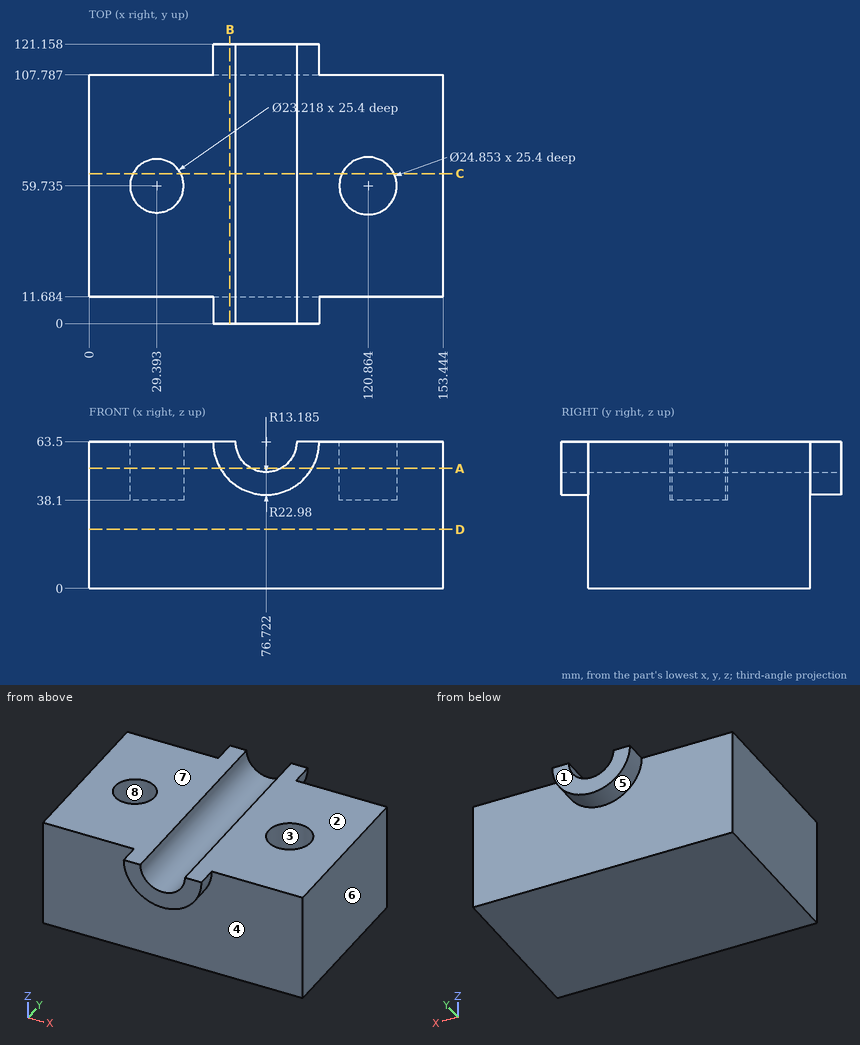
Could you check a few things on this drawing? It's one solid part, dimensions in mm from its lowest x, y, z. A direction names the side the tool comes from. Coordinates: 2 decimals unless noted, no trailing zeros. Write each loop counter-clockwise with the first axis right and the second up, starting at its lowest first coordinate (ties: lowest second). Pieces come first, ordered by that corner, then holes. Notation, with made-up numbers: (-30.75, -4) - (18.25, -4) arc R17 cw to (18.25, 5) - close; hole circle Ø7 at (54, 65.5). An arc over 180 degrees is marked (long way). Return JSON: item names as keys, results as strings. Group by question number.
Item 1: I'm going to push flat-ended pins straight in: pin 1 Ø1 at (y, z) = (35.5, 56) entering from -X; pin 2 Ø8 at (x, z) = (35.5, 25.5) entering from +Y; pin 3 Ø1.5 at (x, z) = (57.5, 38.5) entering from -Y. Where does each tip first touch, or does it pass through?
Item 2: Which directions (+Z, -Z, +X, -X, +Y, -Y) give clear straight access to the entire face, cutting with the end or side of a thin tool? Please do the marked faces 4, 5, 6, 7 and 8.
Item 3: We'd pull the mould along Y, two halves only. Please class the marked faces 1, 2 and 3: pulls with the +Y half, pulls with the -Y half, needs draft (parallel to the pull), parting line crosses it, or undercut.
Item 4: If we section it at A-A (z = 52): Write out the boundary of the cut face in (x, y) (1 decimal), then the cut area to 3 significant figures.
Item 5: If we section it at B-B (x = 61): Write out the boundary of the cut face in (y, z).
Item 6: If we section it at D-D (z = 25.5): Write out the boundary of the cut face in (x, y), then the cut area to 3 significant figures.
Item 7: Please list where these lines run through material, in increasing order: probe 1 along X at (y, z) = (65.5, 40.5) (1 decimal); probe 2 along X at (y, z) = (53.5, 54.5) (1 decimal); probe 3 along X at (y, z) = (50, 61) (1 decimal).
Item 8: If we section it at C-C (y = 65): Write out the boundary of the cut face in (x, z) (1 decimal).
Return value:
{
 "1": {"pin 1": "stops at x = 0", "pin 2": "stops at y = 107.79", "pin 3": "stops at y = 11.68"},
 "2": {"face 4": "-Z, -Y", "face 5": "-Z, +Y", "face 6": "+Z, -Z, +X, +Y, -Y", "face 7": "+Z, +X, -X, +Y, -Y", "face 8": "+Z"},
 "3": {"face 1": "pulls with the +Y half", "face 2": "needs draft", "face 3": "undercut"},
 "4": {"outline": "(0, 11.7) - (56.8, 11.7) - (56.8, 0) - (70.3, 0) - (70.3, 121.2) - (56.8, 121.2) - (56.8, 107.8) - (0, 107.8) - close; (83.2, 0) - (96.6, 0) - (96.6, 11.7) - (153.4, 11.7) - (153.4, 107.8) - (96.6, 107.8) - (96.6, 121.2) - (83.2, 121.2) - close; hole circle Ø23.2 at (29.4, 59.7); hole circle Ø24.9 at (120.9, 59.7)", "area": "13,300 mm^2"},
 "5": {"outline": "(0, 46.74) - (11.68, 46.74) - (11.68, 0) - (107.79, 0) - (107.79, 46.74) - (121.16, 46.74) - (121.16, 63.5) - (0, 63.5) - close"},
 "6": {"outline": "(0, 11.68) - (153.44, 11.68) - (153.44, 107.79) - (0, 107.79) - close", "area": "14,700 mm^2"},
 "7": {"probe 1": "x = 0 to 19.3, 39.5 to 109.9, 131.9 to 153.4", "probe 2": "x = 0 to 19.6, 39.2 to 67.1, 86.4 to 110.1, 131.6 to 153.4", "probe 3": "x = 0 to 23.1, 35.7 to 63.8, 89.7 to 113.1, 128.6 to 153.4"},
 "8": {"outline": "(0, 0) - (153.4, 0) - (153.4, 63.5) - (132.1, 63.5) - (132.1, 38.1) - (109.6, 38.1) - (109.6, 63.5) - (89.9, 63.5) arc R13.2 cw to (63.5, 63.5) - (39.7, 63.5) - (39.7, 38.1) - (19, 38.1) - (19, 63.5) - (0, 63.5) - close"}
}
